from build123d import *

# Parameters (mm, degrees)
CROQUIS1_R                    = 19.05
SALIENTE_EXTRUIR1_DEPTH       = 30
CHAFL_N1_SIZE                 = 2
TALADRO_ROSCADO_1_4_201_D     = 5.1054
TALADRO_ROSCADO_1_4_201_DEPTH = 25
TALADRO_ROSCADO_1_4_201_TIP   = 1.533816902
CHAFL_N2_SIZE                 = 2


with BuildPart() as part:
    # Croquis1 → Saliente-Extruir1 (new body)
    with BuildSketch(Plane(origin=(0, 0, 0), x_dir=(1, 0, 0), z_dir=(0, 1, 0))):
        with Locations(Location((0, 0, 0), (0, 0, 270))):
            Circle(CROQUIS1_R)
    extrude(amount=SALIENTE_EXTRUIR1_DEPTH)

    # Chaflán1
    chafl_n1_edges = [part.edges().sort_by_distance(p)[0] for p in [
        (0, 30, -19.05),
    ]]
    chamfer(chafl_n1_edges, length=CHAFL_N1_SIZE)

    # Taladro roscado 1/4-201
    with Locations(Plane(origin=(0, 30, 0), x_dir=(1, 0, 0), z_dir=(0, 1, 0))):
        with Locations((0, 0)):
            Hole(TALADRO_ROSCADO_1_4_201_D / 2, depth=TALADRO_ROSCADO_1_4_201_DEPTH)
            with Locations((0, 0, -(TALADRO_ROSCADO_1_4_201_DEPTH + TALADRO_ROSCADO_1_4_201_TIP / 2))):  # 118° drill point
                Cone(0, TALADRO_ROSCADO_1_4_201_D / 2, TALADRO_ROSCADO_1_4_201_TIP, mode=Mode.SUBTRACT)

    # Chaflán2
    chafl_n2_edges = [part.edges().sort_by_distance(p)[0] for p in [
        (0, 0, -19.05),
    ]]
    chamfer(chafl_n2_edges, length=CHAFL_N2_SIZE)


solid = part.part
Input: part model. Units: mm. Frame: model coordinates. A direction names the side the tool comes from. Coordinates: 2 decimals unless noted, no trailing zeros. Order: outer loops, then holes, each group sorted by start corner. A loop starts at its lowest first (then second) coordinate and runs counter-clockwise, first axis right, second up. Notation, with made-up numbers: M 88.25,-16.75 L 99.25,-16.75 A21 ccw 99.25,-10.75 Z; hole C 34.5,9 d8. An arc over 180 degrees is marked long. Answer as CSV lines item,"result".
1. First-contact query: P1, Ø1.5, axis at x = 9.5, y = 24.5, coming from the +Z side; P2, Ø3, axis at x = -5, y = 13, coming from the -Z side; P3, Ø6, axis at y = 18.5, z = -4, coming from the +X side. Flat tips, straight axial feed; report the tip coordinate or a pass-through.
Reported:
P1,"z = 16.92"
P2,"z = -18.73"
P3,"x = 19.02"
2. Access query for faces 1 (the cylindrical face through (-2.435, 17.325, -0.767)), 2 (the flat face through (0, 30, 4)). Directions: +Z, -Z, +X, -X, +Y, -Y. A direction counts if a zero-diameter tool reaches every point of the face in a straight line with its end or side. Return the directions, or none.
Reported:
face 1,"+Y"
face 2,"+Z, -Z, +X, -X, +Y"
3. Material intervals for line 1 (Z direction, x = -1, y = 16.5); line 2 (X direction, y = 3.75, z = -12.5); line 3 (Z direction, x = -10, y = 20.5), sorted ascending. Write a range as from..to.
Reported:
line 1,"-19.02..-2.35, 2.35..19.02"
line 2,"-14.38..14.38"
line 3,"-16.21..16.21"
4. Section A-A (y = 14.25). Return the cut outline in (x, z).
Reported:
outline,"C 0,0 d38.1; hole C 0,0 d5.11"
